The listing builds one solid part. Answer for the finished solid, in the listing's coordinates (mm). Face numbers are marked on the shaded views. A direction names the side the tool comes from. Round coordinates to 2 decimals unless told otherwise and drop trailing zeros. Write each loop counter-clockwise with the first axis right and the second up, starting at its lowest first coordinate (ties: lowest second). Pieces come first, ordered by that corner, then holes. Notation, with made-up numbers: M 4.5,38 L 27.5,38 A16 ccw 27.5,69 Z; hole C -8.5,-9.75 d10. An arc over 180 degrees is marked long. Put each result on its own line as item: value. Start each with the question number.
```python
from build123d import *

# Parameters (mm, degrees)
SKETCH_W        = 86
SKETCH_H        = 52
SKETCH_W_2      = 82
SKETCH_H_2      = 48
PAD_DEPTH       = 25
SKETCH005_W     = 86
SKETCH005_H     = 52
PAD003002_DEPTH = 2
SKETCH006_W     = 16
SKETCH006_H     = 16
POCKET_DEPTH    = 2.001


with BuildPart() as part:
    # Sketch → Pad (new body)
    with BuildSketch(Plane.XY):
        with Locations((0, -14)):
            Rectangle(SKETCH_W, SKETCH_H)
        with Locations((0, -14)):
            Rectangle(SKETCH_W_2, SKETCH_H_2, mode=Mode.SUBTRACT)
    extrude(amount=PAD_DEPTH)

    # Sketch005 → Pad003002 (new body)
    with BuildSketch(Plane(origin=(0, 0, 0), x_dir=(1, 0, 0), z_dir=(0, 0, -1))):
        with Locations((0, 14)):
            Rectangle(SKETCH005_W, SKETCH005_H)
    extrude(amount=-PAD003002_DEPTH)

    # Sketch006 → Pocket (cut, through all)
    with BuildSketch(Plane.XY.offset(2)):
        Rectangle(SKETCH006_W, SKETCH006_H)
        with Locations((-25, 0)):
            Rectangle(SKETCH006_W, SKETCH006_H)
        with Locations((25, 0)):
            Rectangle(SKETCH006_W, SKETCH006_H)
    extrude(amount=-POCKET_DEPTH, mode=Mode.SUBTRACT)


solid = part.part
```
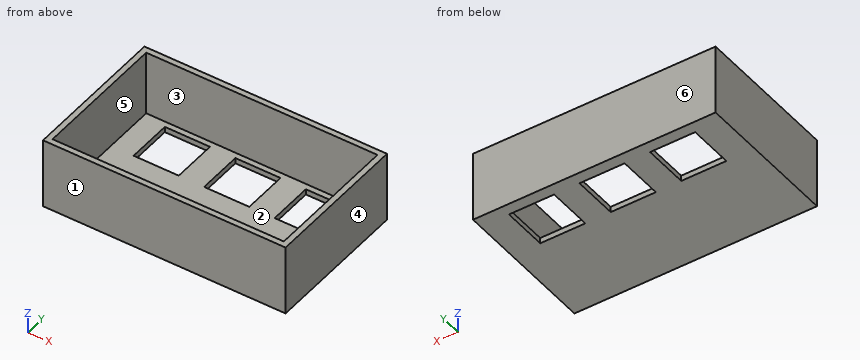
Item 1: Determine the mould class of the marked faces 1, 2, 3 and 4 for opening direction X: released by +X, released by -X, zero draft, split by the parting line, or undercut.
Item 2: Section C-C (y = 2.5) is taken. Give the vertices of the cut face in (x, z), and give its area (3 significant figures).
Item 3: Section B-B (x = 6) is taken. Give the vertices of the cut face in (y, z), and give its area (3 significant figures).
Item 4: Section A-A (z = 9.25) is taken. Give the vertices of the cut face in (x, y).
Item 5: Consider line 1 along Y through (x, z) = (20, 17.5); line 2 along X through (y, z) = (-5.5, 4); line 3 along Z through (x, y) = (-33.5, 3.5). Determine where each line is inside the solid, lowest interval first. Write a range as [from, to].
Item 6: Section D-D (y = -19.5) is taken. Give the vertices of the cut face in (x, z).
Item 7: A flat-ended cylindrical pin translates along its axis: pin 1 (12 mm diameter, centred on x = -0.5, y = -18, fed in from +Z). Find the tip coordinate at first contact, or state that the pin passes through.
Item 8: Which of the six approach directions +Z, -Z, +X, -X, +Y, -Y give full straight-line access (tool end or side, diameter ignored) to the marked faces 5 and 6?
Output values:
1. face 1: zero draft
1. face 2: undercut
1. face 3: undercut
1. face 4: released by +X
2. outline: M -43,0 L -33,0 L -33,2 L -41,2 L -41,25 L -43,25 Z; M -17,0 L -8,0 L -8,2 L -17,2 Z; M 8,0 L 17,0 L 17,2 L 8,2 Z; M 33,0 L 43,0 L 43,25 L 41,25 L 41,2 L 33,2 Z
2. area: 168 mm^2
3. outline: M -40,0 L -8,0 L -8,2 L -38,2 L -38,25 L -40,25 Z; M 8,0 L 12,0 L 12,25 L 10,25 L 10,2 L 8,2 Z
3. area: 164 mm^2
4. outline: M -43,-40 L 43,-40 L 43,12 L -43,12 Z; hole M -41,-38 L 41,-38 L 41,10 L -41,10 Z
5. line 1: y = [-40, -38], [10, 12]
5. line 2: x = [-43, -41], [41, 43]
5. line 3: z = [0, 2]
6. outline: M -43,0 L 43,0 L 43,25 L 41,25 L 41,2 L -41,2 L -41,25 L -43,25 Z
7. pin 1: stops at z = 2
8. face 5: +Z
8. face 6: +Z, -Z, +X, -X, +Y
